Model file for the job. Use its own axes, mm. Face numbers are marked on the shaded views. A direction names the side the tool comes from. Round coordinates to 2 decimals unless told otherwise and drop trailing zeros. Loops run counter-clockwise (first coordinate to the right, second up) from the corner with the lowest first, then second, coordinate; pieces in that order, holes last.
from build123d import *

# Parameters (mm, degrees)
F0_R     = 89.756826
F4_DEPTH = 12.954
F1_R     = 79.193575
F5_DEPTH = 25.4
F2_R     = 67.606004
F6_DEPTH = 35.306
F3_R     = 56.449145
F7_DEPTH = 43.942


with BuildPart() as f4:
    # F0 (on Right) → F4 (new body)
    with BuildSketch(Plane.YZ):
        Circle(F0_R)
    extrude(amount=F4_DEPTH)

    # F1 (on Right) → F5 (join)
    with BuildSketch(Plane.YZ):
        Circle(F1_R)
    extrude(amount=F5_DEPTH)

    # F2 (on Right) → F6 (join)
    with BuildSketch(Plane.YZ):
        Circle(F2_R)
    extrude(amount=F6_DEPTH)

    # F3 (on Right) → F7 (join)
    with BuildSketch(Plane.YZ):
        Circle(F3_R)
    extrude(amount=F7_DEPTH)


solid = f4.part
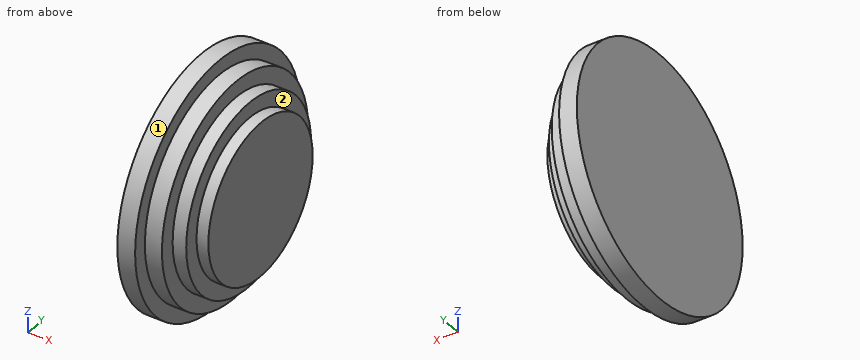
Q1. Slice it at C-C on x = 17. Give the cut face in (y, z), plus the area to 3 significant figures.
Q2. Flat gauge pins, fed straight in: P1, Ø1.5, axis at x = 34, y = -55, coming from the -Z side; P2, Ø3, axis at x = 30, z = 21, coming from the +Y side; P3, Ø1.5, axis at x = 7, y = 66.5, coming from the -Z side. Where does each tip first touch, or does it go through?
Q3. Probe line 1 (X direction, y = 56, z = 47.5); line 2 (X direction, y = 73, z = 40.5); line 3 (Y direction, x = 38, z = 26). List the from-to ranges inside material, lowest first.
Q4. Slice it at D-D on z = 61.5. Give the cut face in (x, y).
Q5. Slice it at A-A on y = 0. Give the cut face in (x, z).
Q6. Tool access for the marked faces 1 and 2: list every direction of +Z, -Z, +X, -X, +Y, -Y with a clear straight run to the whole face (end or side of a thin tool).
Reply:
1. outline: circle Ø158.39 at (0, 0)
1. area: 19,700 mm2
2. P1: stops at z = -40.34
2. P2: stops at y = 64.73
2. P3: stops at z = -61.1
3. line 1: x = 0 to 25.4
3. line 2: x = 0 to 12.95
3. line 3: y = -50.1 to 50.1
4. outline: (0, -65.38) - (12.95, -65.38) - (12.95, -49.89) - (25.4, -49.89) - (25.4, -28.08) - (35.31, -28.08) - (35.31, 28.08) - (25.4, 28.08) - (25.4, 49.89) - (12.95, 49.89) - (12.95, 65.38) - (0, 65.38) - close
5. outline: (0, -89.76) - (12.95, -89.76) - (12.95, -79.19) - (25.4, -79.19) - (25.4, -67.61) - (35.31, -67.61) - (35.31, -56.45) - (43.94, -56.45) - (43.94, 56.45) - (35.31, 56.45) - (35.31, 67.61) - (25.4, 67.61) - (25.4, 79.19) - (12.95, 79.19) - (12.95, 89.76) - (0, 89.76) - close
6. face 1: +X, -X
6. face 2: +X
